```python
from build123d import *

# Parameters (mm, degrees)
SKETCH1_W           = 304.8
SKETCH1_H           = 228.6
BOSS_EXTRUDE1_DEPTH = 12.7
SKETCH7_W           = 112.268
SKETCH7_H           = 12.7
CUT_EXTRUDE2_DEPTH  = 12.7
SKETCH8_W           = 12.7
SKETCH8_H           = 228.6
SKETCH8_W_2         = 3.175
BOSS_EXTRUDE2_DEPTH = 12.7


with BuildPart() as part:
    # Sketch1 → Boss-Extrude1 (new body)
    with BuildSketch(Plane.XY):
        with Locations((152.4, 114.3)):
            Rectangle(SKETCH1_W, SKETCH1_H)
    extrude(amount=BOSS_EXTRUDE1_DEPTH)

    # Sketch7 → Cut-Extrude2 (cut)
    with BuildSketch(Plane.XY.offset(12.7)):
        with Locations((70.358, 222.25)):
            Rectangle(SKETCH7_W, SKETCH7_H)
        with Locations((234.442, 222.25)):
            Rectangle(SKETCH7_W, SKETCH7_H)
        with Locations((70.358, 196.85)):
            Rectangle(SKETCH7_W, SKETCH7_H)
        with Locations((234.442, 196.85)):
            Rectangle(SKETCH7_W, SKETCH7_H)
    extrude(amount=-CUT_EXTRUDE2_DEPTH, mode=Mode.SUBTRACT)

    # Sketch8 → Boss-Extrude2 (add)
    with BuildSketch(Plane.XY.offset(12.7)):
        with Locations((-6.35, 114.3)):
            Rectangle(SKETCH8_W, SKETCH8_H)
        with Locations((306.3875, 114.3)):
            Rectangle(SKETCH8_W_2, SKETCH8_H)
    extrude(amount=-BOSS_EXTRUDE2_DEPTH)


solid = part.part
```
Source: CAD feature listing. Evaluate the final solid. Frame: model axes, mm. A direction names the side the tool comes from. Round coordinates to 2 decimals unless told otherwise and drop trailing zeros. Order: outer loops, then holes, each group sorted by start corner. A loop starts at its lowest first (then second) coordinate and runs counter-clockwise, first axis right, second up. Notation, with made-up numbers: (42.25, 80.5) -> (75.25, 80.5) arc R12 cw to (75.25, 103.5) -> close; hole circle Ø10 at (37, 10). An arc over 180 degrees is marked (long way). One line per item, written item: value. Start each with the question number.
Q1. Pin query (flat end, axial travel): pin 1 (6.5 mm diameter, centred on x = 242.5, z = 7.5, fed in from +Y). Return the tip coordinate at first contact, or that it passes through.
Q2. Access query for faces 1 (the flat face through (290.576, 222, 6)), 2 (the flat face through (178.308, 197, 6)), 3 (the flat face through (145, 0, 6)). Directions: +Z, -Z, +X, -X, +Y, -Y. A direction counts if a zero-diameter tool reaches every point of the face in a straight line with its end or side. Return the directions, or none.
Q3. Draft query along X for faces 4 (the flat face through (307.975, 113, 6)), 5 (the flat face through (152, 228.6, 6)), 6 (the flat face through (70, 190.5, 6)). Return one class per face: pulls with the +X half, pulls with the -X half, needs draft (parallel to the pull), parting line crosses it, or undercut.
Q4. Section query A-A (z = 10.5). Return the cut outline in (x, y) (3 decimals).
Q5. Material intervals for probe 1 along Y at (x, z) = (32, 7), sorted ascending.
Q6. Section query B-B (x = 265.5). Return the cut outline in (y, z).
Findings below:
1. pin 1: y = 215.9
2. face 1: +Z, -Z, +Y
2. face 2: +Z, -Z
2. face 3: +Z, -Z, +X, -X, -Y
3. face 4: pulls with the +X half
3. face 5: needs draft
3. face 6: undercut
4. outline: (-12.7, 0) -> (307.975, 0) -> (307.975, 228.6) -> (290.576, 228.6) -> (290.576, 215.9) -> (178.308, 215.9) -> (178.308, 228.6) -> (126.492, 228.6) -> (126.492, 215.9) -> (14.224, 215.9) -> (14.224, 228.6) -> (-12.7, 228.6) -> close; hole (14.224, 190.5) -> (126.492, 190.5) -> (126.492, 203.2) -> (14.224, 203.2) -> close; hole (178.308, 190.5) -> (290.576, 190.5) -> (290.576, 203.2) -> (178.308, 203.2) -> close
5. probe 1: 0 to 190.5, 203.2 to 215.9
6. outline: (0, 0) -> (190.5, 0) -> (190.5, 12.7) -> (0, 12.7) -> close; (203.2, 0) -> (215.9, 0) -> (215.9, 12.7) -> (203.2, 12.7) -> close
